from build123d import *

# Parameters (mm, degrees)
F0_W        = 135
F0_H        = 25
F1_DEPTH    = 38
F2_W        = 25
F2_H        = 25
F3_DEPTH    = 28
F4_T1_DEPTH = 85


# Not quite as in the source:
# - a fillet or chamfer that OpenCascade refuses, or shapes differently, is made with other operations: its cross-section is extruded or revolved along the edge and cut away or added


with BuildPart() as f1:
    # F0 (on Front) → F1 (new body)
    with BuildSketch(Plane.XZ):
        with Locations((67.5, -12.5)):
            Rectangle(F0_W, F0_H)
    extrude(amount=F1_DEPTH)

    # F2 (on face) → F3 (join)
    with BuildSketch(Plane(origin=(0, 0, 0), x_dir=(-1, 0, 0), z_dir=(0, 1, 0))):
        with Locations((-122.5, -12.5)):
            Rectangle(F2_W, F2_H)
        with Locations((-12.5, -12.5)):
            Rectangle(F2_W, F2_H)
    extrude(amount=F3_DEPTH)

    # F4: fillet of radius 16.8994949366 on 2 edges, made by hand

    # F4_s2 → F4_t1 (cut)
    with BuildSketch(Plane.YZ.offset(25)):
        with BuildLine():
            ThreePointArc((-16.8994949366, 0), (-4.9497474683, -4.9497474683), (0, -16.8994949366))
            Line((0, -16.8994949366), (0, 0))
            Line((0, 0), (-16.8994949366, 0))
        make_face()
        with BuildLine():
            ThreePointArc((-16.8994949366, -25), (-4.9497474683, -20.0502525317), (0, -8.1005050634))
            Line((0, -8.1005050634), (0, -25))
            Line((0, -25), (-16.8994949366, -25))
        make_face()
    extrude(amount=F4_T1_DEPTH, mode=Mode.SUBTRACT)


solid = f1.part
Geometry: final body of the model. Coordinates: model frame, mm. A direction names the side the tool comes from. Give positions to 0.01 mm unless a question says otherwise; leave off trailing zeros. Write each loop counter-clockwise with the first axis right and the second up, starting at its lowest first coordinate (ties: lowest second). Pieces come first, ordered by that corner, then holes.
(1) Ray query, line 1 (X direction, y = 15, z = -18.5); line 2 (Y direction, x = 91.5, z = -5.5); line 3 (Y direction, x = 39, z = -6.75). Return the intervals inside material, ascending.
(2) Access query for faces 1 (the flat face through (123, 28, -12)), 2 (the cylindrical face through (66.905, -6.745, -3.391)). Directions: +Z, -Z, +X, -X, +Y, -Y. A direction counts if a zero-diameter tool reaches every point of the face in a straight line with its end or side. Return the directions, or none.
(3) Cut plane B-B, the plane z = -22.5. Return loops of the section in (x, y).
(4) First-contact query: P1, Ø12, axis at x = 79, z = -19.5, coming from the +Y side; P2, Ø6, axis at x = 86, z = -20, coming from the +Y side. Flat tips, straight axial feed; report the tip coordinate or a pass-through.
(5) Cut plane D-D, the plane y = -6.5. Return loops of the section in (x, z), then the cut area to 3 significant figures.
(6) Cut plane C-C, the plane x = 91. Return loops of the section in (y, z), then the cut area to 3 significant figures.
(7) Cut plane A-A, the plane y = 17. Return loops of the section in (x, z).
(8) Mould query, pull axis X, two halves, no side actions, for faces 3 (the flat face through (0, -5, -13)), 4 (the cylindrical face through (66.905, -6.745, -21.609)), 5 (the flat face through (68, -20, -25)). Classes: released by +X, released by -X, zero draft, split by the parting line, or undercut.
Values follow:
1. line 1: x = 0 to 25, 110 to 135
1. line 2: y = -38 to -4.42
1. line 3: y = -38 to -3.39
2. face 1: +Z, -Z, +X, -X, +Y
2. face 2: +Z, +Y
3. outline: (0, -38) - (135, -38) - (135, 28) - (110, 28) - (110, -8.05) - (25, -8.05) - (25, 28) - (0, 28) - close
4. P1: stops at y = -0.89
4. P2: stops at y = -2.53
5. outline: (0, -25) - (25, -25) - (25, -21.42) - (110, -21.42) - (110, -25) - (135, -25) - (135, 0) - (110, 0) - (110, -3.58) - (25, -3.58) - (25, 0) - (0, 0) - close
5. area: 2,770 mm2
6. outline: (-38, -25) - (-16.9, -25) arc R16.9 ccw to (-0.58, -12.5) arc R16.9 ccw to (-16.9, 0) - (-38, 0) - close
6. area: 829 mm2
7. outline: (0, -25) - (25, -25) - (25, 0) - (0, 0) - close; (110, -25) - (135, -25) - (135, 0) - (110, 0) - close
8. face 3: released by -X
8. face 4: undercut
8. face 5: zero draft
